```python
from build123d import *

# Parameters (mm, degrees)
SKETCH_1_R          = 112.5
EXTRUDE_1_DEPTH     = 1.5
SKETCH_2_R          = 1.6
SKETCH_2_W          = 175.6
SKETCH_2_H          = 130.2
CUT_EXTRUDE_1_DEPTH = 10
FILLET_1_R          = 5
SKETCH_3_R          = 3
CUT_EXTRUDE_2_DEPTH = 10
FILLET_2_R          = 5
CUT_EXTRUDE_3_DEPTH = 10


with BuildPart() as part:
    # 草图1 → 凸台-拉伸1 (new body)
    with BuildSketch(Plane.XY):
        Circle(SKETCH_1_R)
    extrude(amount=EXTRUDE_1_DEPTH)

    # 草图2 → 切除-拉伸1 (cut)
    with BuildSketch(Plane.XY.offset(1.5)):
        with Locations((-13, 68)):
            Circle(SKETCH_2_R)
        with Locations((7, 68)):
            Circle(SKETCH_2_R)
        with Locations((-13, -68)):
            Circle(SKETCH_2_R)
        with Locations((7, -68)):
            Circle(SKETCH_2_R)
        with Locations((24.7, 0)):
            Rectangle(SKETCH_2_W, SKETCH_2_H)
    extrude(amount=-CUT_EXTRUDE_1_DEPTH, mode=Mode.SUBTRACT)

    # 圆角1
    fillet_1_edges = [part.edges().sort_by_distance(p)[0] for p in [
        (91.750967297, 65.1, 0.75),
        (91.750967297, -65.1, 0.75),
    ]]
    fillet(fillet_1_edges, radius=FILLET_1_R)

    # 草图3 → 切除-拉伸2 (cut)
    with BuildSketch(Plane.XY.offset(1.5)):
        with Locations((-63.1, 65.1)):
            Circle(SKETCH_3_R)
        with Locations((-63.1, -65.1)):
            Circle(SKETCH_3_R)
    extrude(amount=-CUT_EXTRUDE_2_DEPTH, mode=Mode.SUBTRACT)

    # 圆角2
    fillet_2_edges = [part.edges().sort_by_distance(p)[0] for p in [
        (-60.1, -65.1, 0.75),
        (-60.1, 65.1, 0.75),
        (-63.1, 62.1, 0.75),
        (-63.1, -62.1, 0.75),
    ]]
    fillet(fillet_2_edges, radius=FILLET_2_R)

    # 草图4 → 切除-拉伸3 (cut)
    with BuildSketch(Plane.XY.offset(1.5)):
        with BuildLine():
            Line((60, 73.1), (70, 73.1))
            ThreePointArc((70, 73.1), (72, 71.1), (70, 69.1))
            Line((70, 69.1), (60, 69.1))
            ThreePointArc((60, 69.1), (58, 71.1), (60, 73.1))
        make_face()
        with BuildLine():
            Line((60, -69.1), (70, -69.1))
            ThreePointArc((70, -69.1), (72, -71.1), (70, -73.1))
            Line((70, -73.1), (60, -73.1))
            ThreePointArc((60, -73.1), (58, -71.1), (60, -69.1))
        make_face()
    extrude(amount=-CUT_EXTRUDE_3_DEPTH, mode=Mode.SUBTRACT)


solid = part.part
```
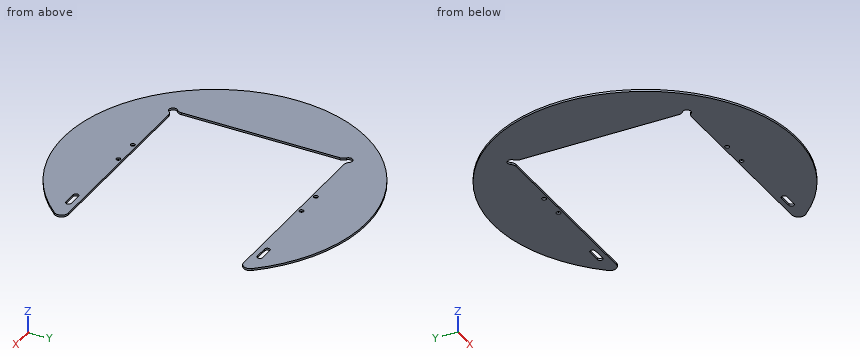
The listing builds one solid part. Answer for the finished solid, in the listing's coordinates (mm). Give positions to 0.01 mm unless a question says otherwise; leave off trailing zeros. Order: outer loops, then holes, each group sorted by start corner. A loop starts at its lowest first (then second) coordinate and runs counter-clockwise, first axis right, second up. Notation, with made-up numbers: M -8,-1 L 51,-1 A27 cw 51,19 Z; hole C -10.75,36.5 d3. An arc over 180 degrees is marked long. Put each result on its own line as item: value. Start each with the question number.
Item 1: The part is cut by section A-A, the plane z = 1. Determine the outline of the cut face in (x, y) (3 decimals).
Item 2: Find the intervals of material crossed by line 1 along X through (y, z) = (67.5, 0.1); line 2 along Y through (x, z) = (7, 1.1); line 3 along X through (y, z) = (-85.5, 0.9), in increasing order.
Item 3: Flat-ended cylindrical pins translate along their axes: P1, Ø5.5, axis at x = -63.1, y = -65.1, coming from the -Z side; P2, Ø0.8, axis at x = 66.5, z = 1, coming from the +Y side. Find the tip coordinate at first contact, or state that the pin passes through.
Item 4: The part is cut by section D-D, the plane y = -15. Determine the outline of the cut face in (x, z).
Item 5: The part is cut by section B-B, the plane x = -41. Determine the outline of the cut face in (y, z), and give its area (3 significant figures).
Item 6: The part is cut by section C-C, the plane x = -21. Determine the outline of the cut face in (y, z).
Answer key:
1. outline: M -64.975,-62.758 A5 ccw -63.1,-58.855 L -63.1,58.855 A5 ccw -64.975,62.758 A3 cw long -60.758,66.975 A5 ccw -56.855,65.1 L 81.5,65.1 A5 ccw 85.291,73.36 A112.5 ccw long 85.291,-73.36 A5 ccw 81.5,-65.1 L -56.855,-65.1 A5 ccw -60.758,-66.975 A3 cw long Z; hole C -13,-68 d3.2; hole C -13,68 d3.2; hole C 7,-68 d3.2; hole C 7,68 d3.2; hole M 60,-73.1 L 70,-73.1 A2 ccw 70,-69.1 L 60,-69.1 A2 ccw Z; hole M 60,69.1 L 70,69.1 A2 ccw 70,73.1 L 60,73.1 A2 ccw Z
2. line 1: x = -90 to -64.9, -61.3 to -14.52, -11.48 to 5.48, 8.52 to 85.77
2. line 2: y = -112.28 to -69.6, -66.4 to -65.1, 65.1 to 66.4, 69.6 to 112.28
2. line 3: x = -73.12 to 73.12
3. P1: passes through
3. P2: stops at y = 91.03
4. outline: M -111.5,0 L -63.1,0 L -63.1,1.5 L -111.5,1.5 Z
5. outline: M -104.76,0 L -65.1,0 L -65.1,1.5 L -104.76,1.5 Z; M 65.1,0 L 104.76,0 L 104.76,1.5 L 65.1,1.5 Z
5. area: 119 mm²
6. outline: M -110.52,0 L -65.1,0 L -65.1,1.5 L -110.52,1.5 Z; M 65.1,0 L 110.52,0 L 110.52,1.5 L 65.1,1.5 Z
